from build123d import *

# Parameters (mm, degrees)
SKETCH_1_W          = 100
SKETCH_1_H          = 87
EXTRUDE_1_DEPTH     = 10
FILLET_1_R          = 10
SKETCH_2_R          = 2.6
CUT_EXTRUDE_1_DEPTH = 10
SKETCH_3_R          = 5
CUT_EXTRUDE_2_DEPTH = 5
SKETCH_4_R          = 3.1
CUT_EXTRUDE_3_DEPTH = 5
CHAMFER_1_SIZE      = 1
CHAMFER_2_SIZE      = 2
SKETCH1_W           = 50
SKETCH1_H           = 40
CUT_EXTRUDE1_DEPTH  = 10
FILLET1_R           = 5


with BuildPart() as part:
    # 草图1 → 凸台-拉伸1 (new body)
    with BuildSketch(Plane.XY):
        Rectangle(SKETCH_1_W, SKETCH_1_H)
    extrude(amount=EXTRUDE_1_DEPTH)

    # 圆角1
    fillet_1_edges = [part.edges().sort_by_distance(p)[0] for p in [
        (50, -43.5, 5),
        (-50, -43.5, 5),
        (-50, 43.5, 5),
        (50, 43.5, 5),
    ]]
    fillet(fillet_1_edges, radius=FILLET_1_R)

    # 草图2 → 切除-拉伸1 (cut)
    with BuildSketch(Plane.XY.offset(10)):
        with Locations((0, 32)):
            Circle(SKETCH_2_R)
        with Locations((-12.7, 32)):
            Circle(SKETCH_2_R)
        with Locations((12.7, 32)):
            Circle(SKETCH_2_R)
        with Locations((-12.7, -32)):
            Circle(SKETCH_2_R)
        with Locations((0, -32)):
            Circle(SKETCH_2_R)
        with Locations((12.7, -32)):
            Circle(SKETCH_2_R)
    extrude(amount=-CUT_EXTRUDE_1_DEPTH, mode=Mode.SUBTRACT)

    # 草图3 → 切除-拉伸2 (cut)
    with BuildSketch(Plane.XY.offset(10)):
        with Locations((-38, 28.5)):
            Circle(SKETCH_3_R)
        with Locations((-38, 0)):
            Circle(SKETCH_3_R)
        with Locations((-38, -28.5)):
            Circle(SKETCH_3_R)
        with Locations((38, -28.5)):
            Circle(SKETCH_3_R)
        with Locations((38, 0)):
            Circle(SKETCH_3_R)
        with Locations((38, 28.5)):
            Circle(SKETCH_3_R)
    extrude(amount=-CUT_EXTRUDE_2_DEPTH, mode=Mode.SUBTRACT)

    # 草图4 → 切除-拉伸3 (cut)
    with BuildSketch(Plane.XY.offset(5)):
        with Locations((-38, 28.5)):
            Circle(SKETCH_4_R)
        with Locations((-38, 0)):
            Circle(SKETCH_4_R)
        with Locations((-38, -28.5)):
            Circle(SKETCH_4_R)
        with Locations((38, 28.5)):
            Circle(SKETCH_4_R)
        with Locations((38, 0)):
            Circle(SKETCH_4_R)
        with Locations((38, -28.5)):
            Circle(SKETCH_4_R)
    extrude(amount=-CUT_EXTRUDE_3_DEPTH, mode=Mode.SUBTRACT)

    # 倒角1
    chamfer_1_edges = [part.edges().sort_by_distance(p)[0] for p in [
        (34.9, 0, 0),
        (34.9, -28.5, 0),
        (-41.1, 28.5, 0),
        (-41.1, 0, 0),
        (-41.1, -28.5, 0),
        (34.9, 28.5, 0),
    ]]
    chamfer(chamfer_1_edges, length=CHAMFER_1_SIZE)

    # 倒角2
    chamfer_2_edges = [part.edges().sort_by_distance(p)[0] for p in [
        (0, 43.5, 10),
        (50, 0, 10),
        (-50, 0, 10),
        (0, -43.5, 10),
        (-47.071067812, -40.571067812, 10),
        (47.071067812, -40.571067812, 10),
        (-47.071067812, 40.571067812, 10),
        (47.071067812, 40.571067812, 10),
    ]]
    chamfer(chamfer_2_edges, length=CHAMFER_2_SIZE)

    # Sketch1 → Cut-Extrude1 (cut)
    with BuildSketch(Plane.XY.offset(10)):
        Rectangle(SKETCH1_W, SKETCH1_H)
    extrude(amount=-CUT_EXTRUDE1_DEPTH, mode=Mode.SUBTRACT)

    # Fillet1
    fillet1_edges = [part.edges().sort_by_distance(p)[0] for p in [
        (25, 20, 5),
        (25, -20, 5),
        (-25, -20, 5),
        (-25, 20, 5),
    ]]
    fillet(fillet1_edges, radius=FILLET1_R)


solid = part.part
For this review, take the finished solid that the model builds, in its own axes (mm). A direction names the side the tool comes from. Coordinates: 2 decimals unless noted, no trailing zeros. Write each loop counter-clockwise with the first axis right and the second up, starting at its lowest first coordinate (ties: lowest second). Pieces come first, ordered by that corner, then holes. Notation, with made-up numbers: (86.5, 78.5) -> (107.5, 78.5) arc R21 ccw to (107.5, 110.5) -> close; hole circle Ø11 at (9, 19). An arc over 180 degrees is marked (long way). Write each question's results on one line, items separated by ' | '. Start each with the question number.
1) Consider section B-B (y = 0). Give the number of separate pieces and of enclosed holes in the cut face, plus the area to 3 significant figures.
2) The part is to be moulded in two halves that separate along X. For faces 1 (the face through (39.67, -25.89, 3.03)), 2 (the face through (22, 20, 0)), 3 (the face through (-46.11, 39.47, 9.46)), say which applies: +X half, -X half, draft (parallel to the pull), parting line (faces both ways), or undercut.
3) Consider section A-A (x = -12.7). Write out the cut boundary in (y, z).
4) For faces 4 (the face through (-43, 0, 8)), 5 (the face through (-23, -19, 5)), 6 (the face through (-47.15, -40.49, 4.06)), list the 3-axis set-ups (+Z, -Z, +X, -X, +Y, -Y) from which the entire face can be reached by the end or side of a thin tool; tool diameter is ignored.
5) Insertion check: pin 1 (4 mm diameter, centred on x = 0, y = -32, fed in from -Z); pin 2 (7 mm diameter, centred on x = 38, y = 0, fed in from -Z); pin 3 (8 mm diameter, centred on x = 38, y = 0, fed in from +Z). Each pin has a flat end and moves straight along its axis. Give the tip position at first contact, or say it passes through.
6) Consider section D-D (x = 7.5). Write out the cut boundary in (y, z), plus the area to 3 significant figures.
7) Wall thickness on L1, parallel to Y at x = -38, z = 2.35; L2, parallel to Y at x = 6.5, z = 8; L3, parallel to Y at x = -12.7, z = 3.25: over which ranges is each line inside the solid? List them lowest first. Write a range as [from, to].
Geometry says:
1) separate pieces: 4 | enclosed holes: 0 | area: 332 mm^2
2) face 1: undercut | face 2: draft | face 3: -X half
3) outline: (-43.5, 0) -> (-34.6, 0) -> (-34.6, 10) -> (-41.5, 10) -> (-43.5, 8) -> close; (-29.4, 0) -> (-20, 0) -> (-20, 10) -> (-29.4, 10) -> close; (20, 0) -> (29.4, 0) -> (29.4, 10) -> (20, 10) -> close; (34.6, 0) -> (43.5, 0) -> (43.5, 8) -> (41.5, 10) -> (34.6, 10) -> close
4) face 4: +Z | face 5: +Z, -Z | face 6: +Z, -Z, -X, -Y
5) pin 1: through | pin 2: z = 0.6 | pin 3: z = 5
6) outline: (-43.5, 0) -> (-20, 0) -> (-20, 10) -> (-41.5, 10) -> (-43.5, 8) -> close; (20, 0) -> (43.5, 0) -> (43.5, 8) -> (41.5, 10) -> (20, 10) -> close | area: 466 mm^2
7) L1: [-43.5, -31.6], [-25.4, -3.1], [3.1, 25.4], [31.6, 43.5] | L2: [-43.5, -20], [20, 43.5] | L3: [-43.5, -34.6], [-29.4, -20], [20, 29.4], [34.6, 43.5]
